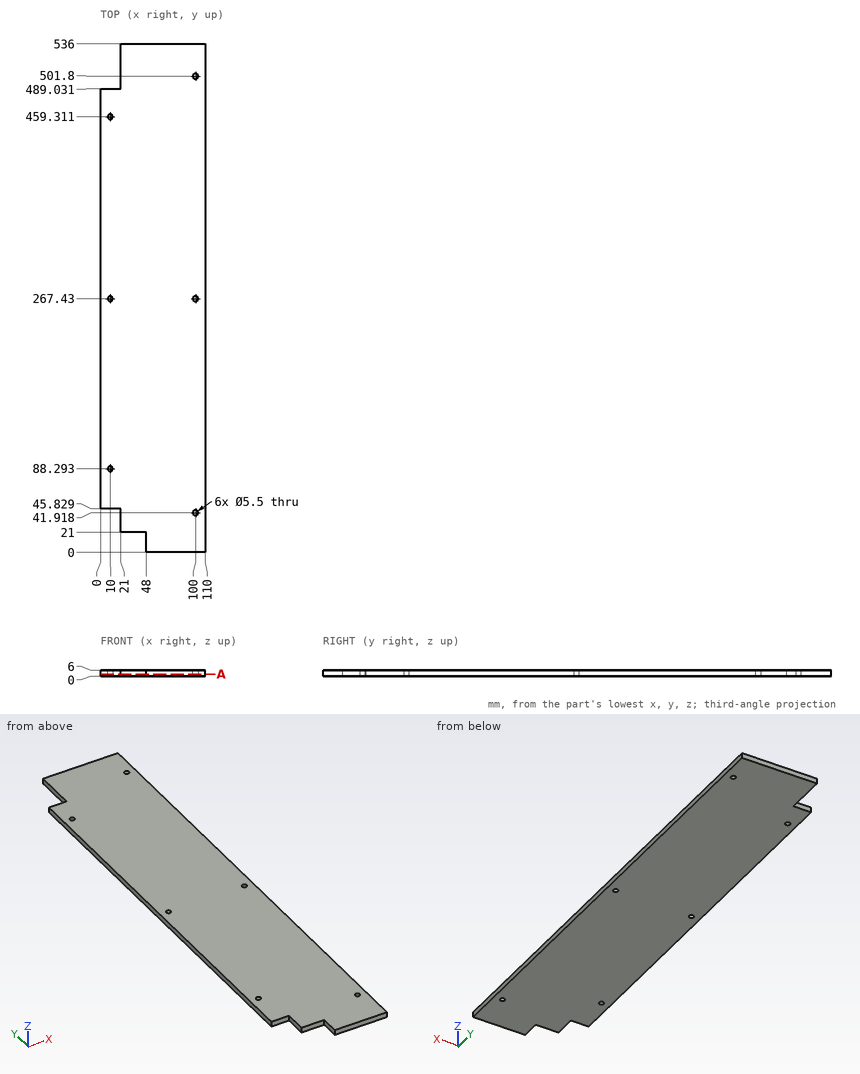
Source: three-view drawing plus pictorial views. Frame: mm from the lowest corner of the part. Give positions to 0.01 mm unless a question says otherwise; leave off trailing zeros. Loops run counter-clockwise (first coordinate to the right, second up) from the corner with the lowest first, then second, coordinate; pieces in that order, holes last. Notation, with made-up numbers: (63, 69) -> (73, 69) arc R23 cw to (73, 93) -> close; hole circle Ø11 at (24, 44). An arc over 180 degrees is marked (long way). Use a Markdown table: item, result. Add a question column.
(1) Ray query, line 1 (Y direction, x = 100, z = 3.75); line 2 (Y direction, x = 10, z = 3.9); line 3 (X direction, y = 502, z = 0.6). Return the intervals inside material, ascending.
(2) Section query A-A (z = 2.05). Output: boundary loops of the cut face in (x, y), then the cut area to 3 significant figures.
(3) First-contact query: pin 1 Ø1.8 at (y, z) = (11, 2.5) entering from -X; pin 2 Ø1.8 at (x, z) = (10.5, 2.5) entering from +Y; pin 3 Ø1.8 at (x, z) = (7.5, 3.5) entering from -Y. Flat tips, straight axial feed; report the tip coordinate or a pass-through.
Checked values:
| question | item | result |
|---|---|---|
| 1 | line 1 | 0 to 39.17, 44.67 to 264.68, 270.18 to 499.05, 504.55 to 536 |
| 1 | line 2 | 45.83 to 85.54, 91.04 to 264.68, 270.18 to 456.56, 462.06 to 489.03 |
| 1 | line 3 | 21 to 97.26, 102.74 to 110 |
| 2 | outline | (0, 45.83) -> (21, 45.83) -> (21, 21) -> (48, 21) -> (48, 0) -> (110, 0) -> (110, 536) -> (21, 536) -> (21, 489.03) -> (0, 489.03) -> close; hole circle Ø5.5 at (10, 88.29); hole circle Ø5.5 at (10, 267.43); hole circle Ø5.5 at (10, 459.31); hole circle Ø5.5 at (100, 41.92); hole circle Ø5.5 at (100, 267.43); hole circle Ø5.5 at (100, 501.8) |
| 2 | area | 56,300 mm^2 |
| 3 | pin 1 | x = 48 |
| 3 | pin 2 | y = 489.03 |
| 3 | pin 3 | y = 45.83 |
